Can you work these out from the model? Positions are in its coordinate system, mm. A direction names the side the tool comes from. Coordinates: 2 decimals unless noted, no trailing zeros. Order: outer loops, then holes, each group sorted by start corner. A loop starts at its lowest first (then second) coordinate and runs counter-clockwise, first axis right, second up. Notation, with made-up numbers: (25.25, 85.5) -> (64.25, 85.5) arc R25 cw to (64.25, 114.5) -> close; hole circle Ø5 at (-38.5, 47.5). An arc over 180 degrees is marked (long way). Return JSON: item names as keys, results as strings. Group by question number.
1) For pin 1 (2 mm diameter, centred on x = 6, z = -1.5, fed in from +Y); pin 2 (2 mm diameter, centred on x = -4.5, z = 1, fed in from -Y), each with a flat end and sliding along its axis, tell me the tip position at first contact or that it passes through.
2) If we section it at D-D, the plane x = 0: Please give me the cut outline in (y, z).
3) For faces 1 (the flat face through (-2, 9.678, -2)), 2 (the flat face through (-1, 6.928, 3)), which set-ups out of +Z, -Z, +X, -X, +Y, -Y let a thin tool reach every point of the face, with its end or its side?
4) If we section it at B-B, the plane x = -5.5: Please give me the cut outline in (y, z), then the cut area to 3 significant figures.
5) If we section it at C-C, the plane z = -3: Please give me the cut outline in (x, y).
6) If I drill on probe 1 along X at (y, z) = (0, 0.25); probe 2 along Y at (x, z) = (5.25, 0.5); probe 3 along X at (y, z) = (-2.25, 0), over which ranges is the centre line in solid material (lowest first)? Write a range as from..to.
7) If we section it at A-A, the plane y = 0: Please give me the cut outline in (x, z), then the cut area to 3 significant figures.
8) Thinking about a two-plate mould opening in Y: for faces 3 (the flat face through (5.3, 8.6, 0.1)), 4 (the cylindrical face through (0, -8, 0)), 5 (the flat face through (0, 7.2, -4)), which applies, +Y half, -Y half, draft (parallel to the pull), parting line (faces both ways), or undercut?
from build123d import *

# Parameters (mm, degrees)
BOSS_EXTRUDE1_DEPTH = 4
FILLET2_R           = 1
FILLET3_R           = 1


with BuildPart() as part:
    # Sketch1 → Boss-Extrude1 (new, symmetric)
    with BuildSketch(Plane.XY):
        with BuildLine():
            Line((-4, 9.67820323), (4, 9.67820323))
            Line((4, 9.67820323), (6.391333959, 7.690958992))
            ThreePointArc((6.391333959, 7.690958992), (0, -10), (-6.391333959, 7.690958992))
            Line((-6.391333959, 7.690958992), (-4, 9.67820323))
        make_face()
        with BuildLine():
            Line((-4, 6.92820323), (4, 6.92820323))
            ThreePointArc((4, 6.92820323), (0, -8), (-4, 6.92820323))
        make_face(mode=Mode.SUBTRACT)
    extrude(amount=BOSS_EXTRUDE1_DEPTH, both=True)

    # Sketch2 → Cut-Revolve1 (revolve, cut)
    with BuildSketch(Plane.XY):
        with BuildLine():
            Line((0, 6.72820323), (0, 11.87820323))
            ThreePointArc((0, 11.87820323), (1.886484437, 10.810093892), (1.941176471, 8.642909113))
            ThreePointArc((1.941176471, 8.642909113), (1.761207875, 8.175401262), (1.7, 7.67820323))
            Line((1.7, 7.67820323), (1.7, 6.72820323))
            Line((1.7, 6.72820323), (0, 6.72820323))
        make_face()
    revolve(axis=Axis((0, 6.72820323, 0), (0, 1, 0)), mode=Mode.SUBTRACT)

    # Fillet2
    # the kernel refuses this fillet: 1 mm, written as the material it takes off along each edge
    with BuildSketch(Plane(origin=(0, 6.92820323, 0), x_dir=(1, 0, 0), z_dir=(0, 0, -1))) as fillet2_piece_1:
        with BuildLine():
            CenterArc((2.730196097, -1), FILLET2_R, 90, 103.774146998)
            Line((1.758954285, -1.238095238), (1.661830104, -1.261904762))
            ThreePointArc((1.661830104, -1.261904762), (1.6, -0.75), (1.6, 0))
            Line((1.6, 0), (1.7, 0.1))
            Line((1.7, 0.1), (2.730196097, 0.1))
            Line((2.730196097, 0.1), (2.730196097, 0))
        make_face()
    revolve(axis=Axis((0, 6.92820323, 0), (0, -1, 0)), mode=Mode.SUBTRACT)

    # Fillet3
    fillet3_edges = [part.edges().sort_by_distance(p)[0] for p in [
        (-4, 6.92820323, 0),
        (4, 6.92820323, 0),
        (-4, 9.67820323, 0),
        (4, 9.67820323, 0),
    ]]
    fillet(fillet3_edges, radius=FILLET3_R)


solid = part.part
Result sheet:
{
 "1": {"pin 1": "stops at y = 8.85", "pin 2": "stops at y = -9.37"},
 "2": {"outline": "(-10, -4) -> (-8, -4) -> (-8, 4) -> (-10, 4) -> close; (6.93, -4) -> (9.68, -4) -> (9.68, -2.2) arc R2.2 cw to (8.64, -1.94) arc R2.05 ccw to (8.17, -1.76) arc R1 ccw to (6.93, -2.73) -> close; (6.93, 2.73) arc R1 ccw to (8.17, 1.76) arc R2.05 ccw to (8.64, 1.94) arc R2.2 cw to (9.68, 2.2) -> (9.68, 4) -> (6.93, 4) -> close"},
 "3": {"face 1": "+Z, -Z, +X, -X, +Y", "face 2": "+Z, -Z"},
 "4": {"outline": "(-8.35, -4) -> (-5.81, -4) -> (-5.81, 4) -> (-8.35, 4) -> close; (5.81, -4) -> (8.43, -4) -> (8.43, 4) -> (5.81, 4) -> close", "area": "41.3 mm2"},
 "5": {"outline": "(-6.39, 7.69) arc R10 ccw (long way) to (6.39, 7.69) -> (4.28, 9.45) arc R1 ccw to (3.64, 9.68) -> (-3.64, 9.68) arc R1 ccw to (-4.28, 9.45) -> close; hole (-4.25, 6.78) arc R8 ccw (long way) to (4.25, 6.78) arc R1 ccw to (3.72, 6.93) -> (-3.72, 6.93) arc R1 ccw to start"},
 "6": {"probe 1": "x = -10..-8, 8..10", "probe 2": "y = -8.51..-6.04, 6.04..8.64", "probe 3": "x = -9.74..-7.68, 7.68..9.74"},
 "7": {"outline": "(-10, -4) -> (-8, -4) -> (-8, 4) -> (-10, 4) -> close; (8, -4) -> (10, -4) -> (10, 4) -> (8, 4) -> close", "area": "32.0 mm2"},
 "8": {"face 3": "+Y half", "face 4": "undercut", "face 5": "draft"}
}
